Geometry: see drawing. Coordinates: mm, zero at the bounding-box minimum. A direction names the side the tool comes from. Give positions to 0.01 mm unless a question says otherwise; leave off trailing zeros. Loops run counter-clockwise (first coordinate to the right, second up) from the corner with the lowest first, then second, coordinate; pieces in that order, holes last. Notation, with made-up numbers: (25.5, 3) - (69.5, 3) arc R15 cw to (69.5, 25) - close; hole circle Ø4 at (43.25, 87). An arc over 180 degrees is marked (long way). Use one line per item in the form item = value.
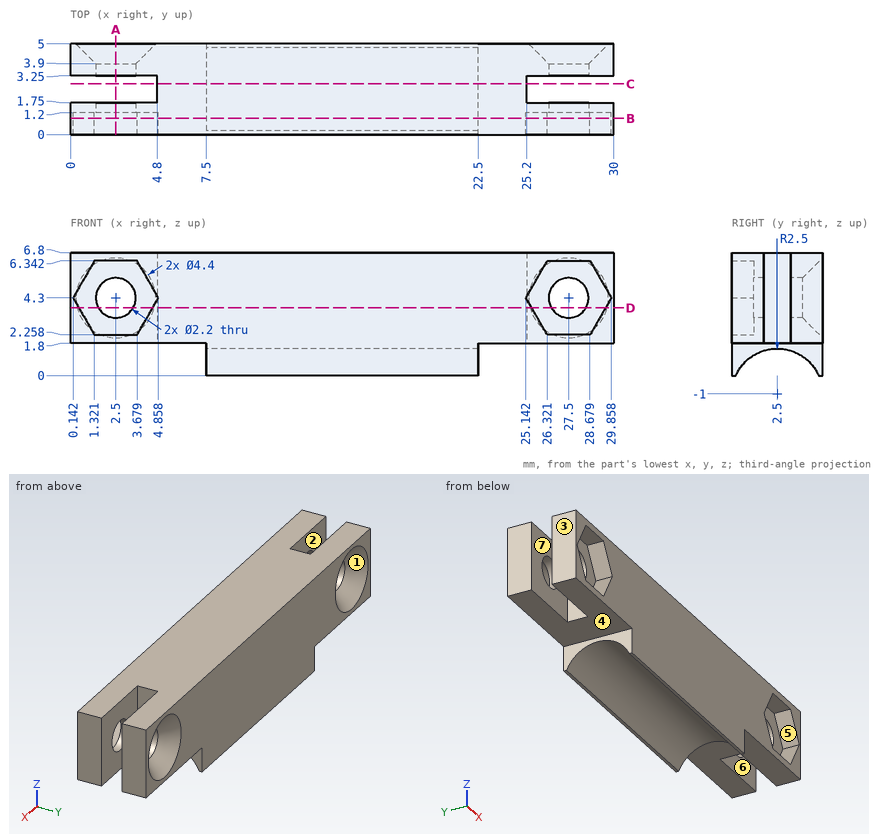
(1) Pull-direction query (Y, two-part tool) for the marked faces 1, 2 and 3; classes: released by +Y, released by -Y, zero draft, split by the parting line, or undercut.
Solution:
face_1 = released by +Y
face_2 = undercut
face_3 = zero draft
(2) Cut plane D-D (z = 3.75). Give the number of separate pieces and of enclosed holes in the cut face, plus the area to 3 significant figures.
Solution:
separate_pieces = 5
enclosed_holes = 0
area = 114 mm2
(3) Cut plane A-A (x = 2.5). Return the cut outline in (y, z).
Solution:
outline = (0, 1.8) - (1.75, 1.8) - (1.75, 3.2) - (1.2, 3.2) - (1.2, 2.26) - (0, 2.26) - close; (0, 6.34) - (1.2, 6.34) - (1.2, 5.4) - (1.75, 5.4) - (1.75, 6.8) - (0, 6.8) - close; (3.25, 1.8) - (5, 1.8) - (5, 2.1) - (3.9, 3.2) - (3.25, 3.2) - close; (3.25, 5.4) - (3.9, 5.4) - (5, 6.5) - (5, 6.8) - (3.25, 6.8) - close
(4) Access query for the marked faces 4, 5, 6 and 7. Directions: +Z, -Z, +X, -X, +Y, -Y. A direction counts if a zero-diameter tool reaches every point of the face in a straight line with its end or side. Return the directions, or none.
Solution:
face_4 = -Z, -X, +Y, -Y
face_5 = -Y
face_6 = +Z, -Z, +X
face_7 = +Z, -Z, -X
(5) Cut plane C-C (y = 2.8). Return the cut outline in (x, z), plus the area to 3 significant figures.
Solution:
outline = (4.8, 1.8) - (7.5, 1.8) - (7.5, 1.48) - (22.5, 1.48) - (22.5, 1.8) - (25.2, 1.8) - (25.2, 6.8) - (4.8, 6.8) - close
area = 107 mm2
(6) Cut plane B-B (y = 0.9). Return the cut outline in (x, z).
Solution:
outline = (0, 1.8) - (7.5, 1.8) - (7.5, 0.92) - (22.5, 0.92) - (22.5, 1.8) - (30, 1.8) - (30, 6.8) - (0, 6.8) - close; hole (0.14, 4.3) - (1.32, 2.26) - (3.68, 2.26) - (4.86, 4.3) - (3.68, 6.34) - (1.32, 6.34) - close; hole (25.14, 4.3) - (26.32, 2.26) - (28.68, 2.26) - (29.86, 4.3) - (28.68, 6.34) - (26.32, 6.34) - close
(7) Material intervals for L1, parallel to Z at x = 2.5, y = 3.75; L2, parallel to Y at x = 4, z = 6.25; L3, parallel to Z at x = 6.5, y = 4.6, sorted ascending. Write a range as from..to.
Solution:
L1 = 1.8..3.2, 5.4..6.8
L2 = 0..1.75, 3.25..5
L3 = 1.8..6.8
(8) Pin query (flat end, axial travel): P1, Ø0.6, axis at x = 27.5, y = 1, coming from the -Z side; P2, Ø2.5, axis at x = 2.5, z = 4.3, coming from the +Y side; P3, Ø3, axis at x = 27.5, z = 4.3, coming from the -Y side. Return the tip coordinate at first contact, or that it passes through.
Solution:
P1 = 1.8
P2 = 4.05
P3 = 1.2
